Can you work these out from the model? Positions are in its coordinate system, mm. A direction names the side the tool comes from. Give positions to 0.01 mm unless a question says otherwise; leave off trailing zeros. Write each loop counter-clockwise with the first axis right and the second up, starting at its lowest first coordinate (ties: lowest second). Pieces come first, ordered by that corner, then holes. Notation, with made-up numbers: (32.5, 5) -> (36.5, 5) arc R34 ccw to (36.5, 39) -> close; hole circle Ø5 at (72, -2.75). An arc over 180 degrees is marked (long way). Answer as CSV lines item,"result". Start each with the question number.
1. If we mould it in two halves opening along Y, with no side actions, what happens to faces 5 (the face through (-5.229, -12.834, -17.255)), 6 (the face through (0, 0, 25)), 7 (the face through (-5.38, 12.77, -17.26))? For each: pulls with the +Y half, pulls with the -Y half, needs draft (parallel to the pull), parting line crosses it, or undercut.
2. If we section it at A-A on z = -12.5: Write out the boundary of the cut face in (x, y), plus the area to 3 significant figures.
3. On a 3-axis mill with a long thin cutter (end or side, diameter ignored), from which of +Z, -Z, +X, -X, +Y, -Y can I reach the whole of each face in a straight line? I mean faces 1 (the face through (5.38, -12.77, -17.26)), 2 (the face through (-12.834, 5.229, -17.255)), 3 (the face through (12.77, 5.38, -17.26)), 4 (the face through (11.923, 3.755, 37.675)). Say none if no direction works.
4. If we section it at D-D on y = 16.5: Write out the boundary of the cut face in (x, z), plus the area to 3 significant figures.
5. I need wall thicknesses on line 1 (Y direction, x = 0, z = 35); line 2 (Z direction, x = 20, y = 20); line 3 (Z direction, x = -9, y = 7). Which ranges of each line are inside material? Lowest first, please. Write a range as [from, to].
6. I'm going to push flat-ended pins straight in: P1, Ø20, axis at x = -1, y = -2, coming from the +Z side; P2, Ø6, axis at x = -11, z = -8, coming from the -Y side; P3, Ø12, axis at y = -14, z = -12, coming from the +X side. Where does each tip first touch, or does it pass through?
7. If we section it at C-C on x = 9.5: Write out the boundary of the cut face in (y, z), plus the area to 3 significant figures.
8. If we section it at B-B on y = -8: Write out the boundary of the cut face in (x, z), plus the area to 3 significant figures.
```python
from build123d import *

# Parameters (mm, degrees)
F0_W     = 50
F0_H     = 50
F1_DEPTH = 50
F2_R     = 12.5
F3_DEPTH = 25
F5_DEPTH = 35


with BuildPart() as f1:
    # F0 (on Top) → F1 (new body)
    with BuildSketch(Plane.XY):
        Rectangle(F0_W, F0_H)
    extrude(amount=F1_DEPTH)

    # F2 (on face) → F3 (cut)
    with BuildSketch(Plane.XY.offset(50)):
        Circle(F2_R)
    extrude(amount=-F3_DEPTH, mode=Mode.SUBTRACT)

    # F4 (on face) → F5 (join)
    with BuildSketch(Plane(origin=(0, 0, 0), x_dir=(1, 0, 0), z_dir=(0, 0, -1))):
        Polygon((0, 15), (-10.606602, 10.606602), (-15, 0), (-10.606602, -10.606602), (0, -15), (10.606602, -10.606602), (15, 0), (10.606602, 10.606602), align=None)
    extrude(amount=F5_DEPTH)


solid = f1.part
```
Computed values:
1,face 5,"pulls with the -Y half"
1,face 6,"undercut"
1,face 7,"pulls with the +Y half"
2,outline,"(-15, 0) -> (-10.61, -10.61) -> (0, -15) -> (10.61, -10.61) -> (15, 0) -> (10.61, 10.61) -> (0, 15) -> (-10.61, 10.61) -> close"
2,area,"636 mm2"
3,face 1,"-Z, +X, -Y"
3,face 2,"-Z, -X, +Y"
3,face 3,"-Z, +X, +Y"
3,face 4,"+Z"
4,outline,"(-25, 0) -> (25, 0) -> (25, 50) -> (-25, 50) -> close"
4,area,"2,500 mm2"
5,line 1,"y = [-25, -12.5], [12.5, 25]"
5,line 2,"z = [0, 50]"
5,line 3,"z = [-35, 25]"
6,P1,"stops at z = 25"
6,P2,"stops at y = -11.69"
6,P3,"stops at x = 11.69"
7,outline,"(-25, 0) -> (-11.06, 0) -> (-11.06, -35) -> (11.06, -35) -> (11.06, 0) -> (25, 0) -> (25, 50) -> (8.12, 50) -> (8.12, 25) -> (-8.12, 25) -> (-8.12, 50) -> (-25, 50) -> close"
7,area,"2,870 mm2"
8,outline,"(-25, 0) -> (-11.69, 0) -> (-11.69, -35) -> (11.69, -35) -> (11.69, 0) -> (25, 0) -> (25, 50) -> (9.6, 50) -> (9.6, 25) -> (-9.6, 25) -> (-9.6, 50) -> (-25, 50) -> close"
8,area,"2,840 mm2"
